Geometry: final body of the model. Coordinates: model frame, mm. A direction names the side the tool comes from. Round coordinates to 2 decimals unless told otherwise and drop trailing zeros. Loops run counter-clockwise (first coordinate to the right, second up) from the corner with the lowest first, then second, coordinate; pieces in that order, holes last. Notation, with made-up numbers: (80.25, 17) - (121.25, 17) arc R30 ccw to (121.25, 40) - close; hole circle Ø1 at (4, 3.25). An arc over 180 degrees is marked (long way). Return JSON: item names as keys, results as strings. Group by question number.
1. Section D-D on x = 6.5. Return loops of the section in (y, z), and give its area (3 significant figures).
2. Section A-A on y = 23. Return loops of the section in (x, z).
3. Set-up query: faces 5 (the face through (50, 3, -19)), 6 (the face through (32, 15, 20)), 7 (the face through (38, 1, -20)). Return all of +Z, -Z, +X, -X, +Y, -Y with unobstructed straight access to the full face (end or side cutting, diameter ignored); none if empty.
4. Draft query along Z for faces 1 (the face through (-1, -2, 0)), 2 (the face through (-75.07, -0.99, 23)), 3 (the face through (34, 15, 19)), 4 (the face through (75.07, -0.99, -23)). Return one class per face: +Z half, -Z half, draft (parallel to the pull), parting line (faces both ways), or undercut.
5. Section B-B on x = 47.5. Return loops of the section in (y, z).
6. First-contact query: pin 1 Ø1.2 at (y, z) = (20.5, -20) entering from +X; pin 2 Ø12 at (y, z) = (15.5, -17.5) entering from -X; pin 3 Ø3 at (x, z) = (14, -19) entering from +Y. Flat tips, straight axial feed; report the tip coordinate or a pass-through.
7. Material intervals for probe 1 along Y at (x, z) = (-5.5, 20.5), sorted ascending.
8. Section C-C on z = -4. Return loops of the section in (x, y).
from build123d import *

# Parameters (mm, degrees)
EXTRUDE_3_DEPTH     = 2
CUT_EXTRUDE_START   = -3
SKETCH_4_W          = 2.2
SKETCH_4_H          = 6.2
CUT_EXTRUDE_2_DEPTH = 4
EXTRUDE_4_DEPTH     = 2.5
FILLET_1_R          = 5


with BuildPart() as part:
    # Эскиз1 → Бобышка-Вытянуть3 (new body)
    with BuildSketch(Plane(origin=(0, 0, 0), x_dir=(1, 0, 0), z_dir=(0, 1, 0))):
        with BuildLine():
            Line((71.5, 24.5), (-71.5, 24.5))
            ThreePointArc((-71.5, 24.5), (-75.035533906, 23.035533906), (-76.5, 19.5))
            Line((-76.5, 19.5), (-76.5, -19.5))
            ThreePointArc((-76.5, -19.5), (-75.035533906, -23.035533906), (-71.5, -24.5))
            Line((-71.5, -24.5), (71.5, -24.5))
            ThreePointArc((71.5, -24.5), (75.035533906, -23.035533906), (76.5, -19.5))
            Line((76.5, -19.5), (76.5, 19.5))
            ThreePointArc((76.5, 19.5), (75.035533906, 23.035533906), (71.5, 24.5))
        make_face()
    extrude(amount=-EXTRUDE_3_DEPTH)

    # Эскиз4 → Вырез-Вытянуть2 (cut)
    with BuildSketch(Plane(origin=(0, 0, 0), x_dir=(1, 0, 0), z_dir=(0, 1, 0)).offset(CUT_EXTRUDE_START)):
        with Locations((-75.4, -11.1)):
            Rectangle(SKETCH_4_W, SKETCH_4_H)
    cut_extrude_2 = extrude(amount=CUT_EXTRUDE_2_DEPTH, mode=Mode.SUBTRACT)

    # Зеркальное отражение3: Вырез-Вытянуть2 across plane
    add(cut_extrude_2.mirror(Plane.XY), mode=Mode.SUBTRACT)

    # Эскиз6 → Бобышка-Вытянуть4 (add)
    with BuildSketch(Plane(origin=(0, 0, -21.5), x_dir=(-1, 0, 0), z_dir=(0, 0, -1))):
        with BuildLine():
            ThreePointArc((-36, 28.6), (-35.589949494, 29.589949494), (-34.6, 30))
            Line((-34.6, 30), (-33.4, 30))
            ThreePointArc((-33.4, 30), (-32.410050506, 29.589949494), (-32, 28.6))
            Line((-32, 28.6), (-32, 0))
            Line((-32, 0), (-36, 0))
            Line((-36, 0), (-36, 28.6))
        make_face()
        with BuildLine():
            ThreePointArc((-50.4, 8), (-49.410050506, 7.589949494), (-49, 6.6))
            Line((-49, 6.6), (-49, 0))
            Line((-49, 0), (-52, 0))
            Line((-52, 0), (-52, 6.6))
            ThreePointArc((-52, 6.6), (-51.589949494, 7.589949494), (-50.6, 8))
            Line((-50.6, 8), (-50.4, 8))
        make_face()
    extrude_4 = extrude(amount=-EXTRUDE_4_DEPTH)

    # Зеркальное отражение4: Бобышка-Вытянуть4 across plane
    add(extrude_4.mirror(Plane.XY))

    # Скругление1
    fillet_1_edges = [part.edges().sort_by_distance(p)[0] for p in [
        (36, 0, 20.25),
        (49, 0, 20.25),
        (36, 0, -20.25),
        (49, 0, -20.25),
    ]]
    fillet(fillet_1_edges, radius=FILLET_1_R)


solid = part.part
Taken from the geometry:
{
 "1": {"outline": "(-2, -24.5) - (0, -24.5) - (0, 24.5) - (-2, 24.5) - close", "area": "98.0 mm2"},
 "2": {"outline": "(32, -21.5) - (36, -21.5) - (36, -19) - (32, -19) - close; (32, 19) - (36, 19) - (36, 21.5) - (32, 21.5) - close"},
 "3": {"face 5": "+X, -X, +Y", "face 6": "+Z, -Z, -X, +Y", "face 7": "+Z, -Z, +Y"},
 "4": {"face 1": "draft", "face 2": "+Z half", "face 3": "undercut", "face 4": "-Z half"},
 "5": {"outline": "(-2, -24.5) - (0, -24.5) - (0, -21.5) - (1.43, -21.5) - (1.43, -19) - (0, -19) - (0, 19) - (1.43, 19) - (1.43, 21.5) - (0, 21.5) - (0, 24.5) - (-2, 24.5) - close"},
 "6": {"pin 1": "x = 36", "pin 2": "x = 32", "pin 3": "y = 0"},
 "7": {"probe 1": "-2 to 0"},
 "8": {"outline": "(-76.5, -2) - (76.5, -2) - (76.5, 0) - (-76.5, 0) - close"}
}
